Verification items for this drawing (mm, ordinates from the low corner). Coordinates: 2 decimals unless noted, no trailing zeros. Order: outer loops, then holes, each group sorted by start corner. A loop starts at its lowest first (then second) coordinate and runs counter-clockwise, first axis right, second up. Notation, with made-up numbers: M -11.5,84 L -5.5,84 A21 ccw -5.5,103 Z; hole C -33.5,30 d9. An arc over 180 degrees is marked long. Answer as a JSON object with one key per item and string values. Group by question number.
(1) Cross-section at A-A (y = 26.5). Enter the section's corners in (x, z).
(2) Cross-section at D-D (x = 6.5). Enter the section's corners in (y, z).
(3) Cross-section at B-B (z = 1). Enter the section's corners in (x, y), plus the area to 3 significant figures.
(4) Material ranges on line 1 (X direction, y = 24.5, z = 0.4); line 2 (X direction, y = 22.25, z = 1.9); line 3 (Y direction, x = 44, z = 2.1), recorded low to high.
(5) Cross-section at C-C (x = 34). Enter the section's corners in (y, z), plus the area to 3 significant figures.
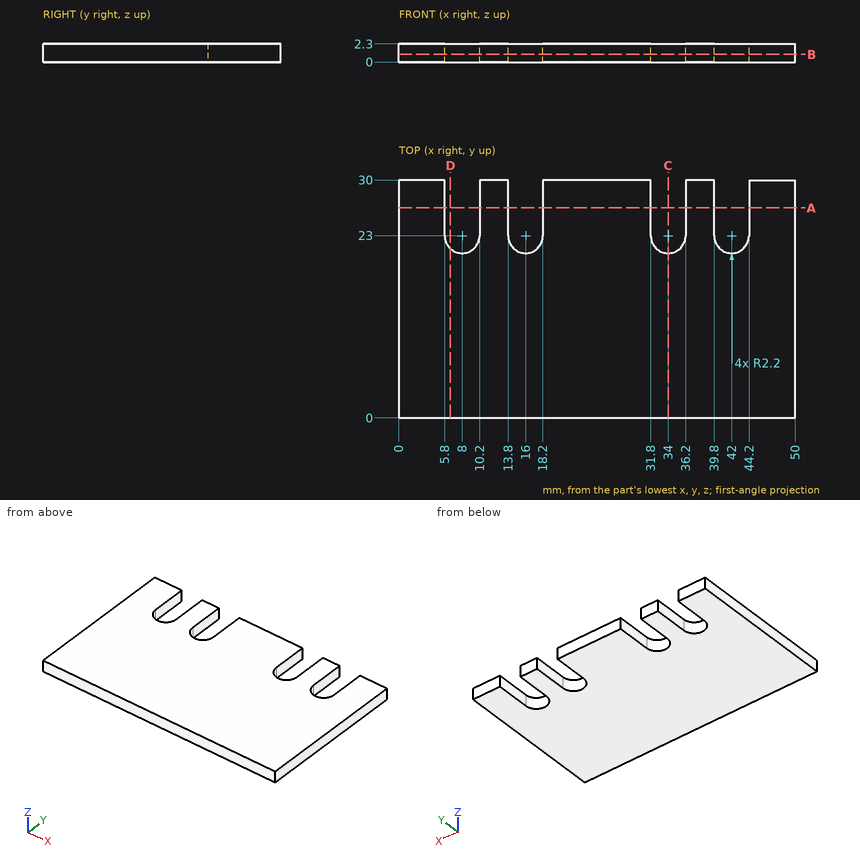
Taken from the geometry:
{
 "1": {"outline": "M 0,0 L 5.8,0 L 5.8,2.3 L 0,2.3 Z; M 10.2,0 L 13.8,0 L 13.8,2.3 L 10.2,2.3 Z; M 18.2,0 L 31.8,0 L 31.8,2.3 L 18.2,2.3 Z; M 36.2,0 L 39.8,0 L 39.8,2.3 L 36.2,2.3 Z; M 44.2,0 L 50,0 L 50,2.3 L 44.2,2.3 Z"},
 "2": {"outline": "M 0,0 L 21.39,0 L 21.39,2.3 L 0,2.3 Z"},
 "3": {"outline": "M 0,0 L 50,0 L 50,30 L 44.2,30 L 44.2,23 A2.2 cw 39.8,23 L 39.8,30 L 36.2,30 L 36.2,23 A2.2 cw 31.8,23 L 31.8,30 L 18.2,30 L 18.2,23 A2.2 cw 13.8,23 L 13.8,30 L 10.2,30 L 10.2,23 A2.2 cw 5.8,23 L 5.8,30 L 0,30 Z", "area": "1,350 mm²"},
 "4": {"line 1": "x = 0 to 5.8, 10.2 to 13.8, 18.2 to 31.8, 36.2 to 39.8, 44.2 to 50", "line 2": "x = 0 to 5.93, 10.07 to 13.93, 18.07 to 31.93, 36.07 to 39.93, 44.07 to 50", "line 3": "y = 0 to 22.08"},
 "5": {"outline": "M 0,0 L 20.8,0 L 20.8,2.3 L 0,2.3 Z", "area": "47.8 mm²"}
}
